For this review, use the dimensioned drawing (mm, ordinates from the lowest corner) and the shaded views. Coordinates: 2 decimals unless noted, no trailing zeros. Loops run counter-clockwise (first coordinate to the right, second up) from the corner with the lowest first, then second, coordinate; pieces in that order, holes last. Notation, with made-up numbers: (-4.75, -19) - (25.25, -19) arc R15 cw to (25.25, 0) - close; hole circle Ø5 at (42, -37). An arc over 180 degrees is marked (long way). Use a Markdown table: item, result. Add a question column.
1) Add section C-C, the plane y = 3.75. Give the boundary of the cut face in (x, z), and give its area (3 significant figures).
2) Add section A-A, the plane x = 44. Give the boundary of the cut face in (y, z), and give its area (3 significant figures).
3) The part is to be moulded in two halves that separate along Z. For the marked faces 1, 2 and 3, say which applies: pulls with the +Z half, pulls with the -Z half, needs draft (parallel to the pull), parting line crosses it, or undercut.
4) To check wall thickness, follow L1, parallel to X at y = 7.25, z = 9.75; L2, parallel to Z at x = 36, y = 3.5; L3, parallel to Z at x = 44, y = 3. State the ranges of each line that lie inside material, in increasing order. Write a range as [from, to].
5) Add section B-B, the plane z = 10. Give the boundary of the cut face in (x, y).
6) Add section D-D, the plane z = 6.5. Give the boundary of the cut face in (x, y).
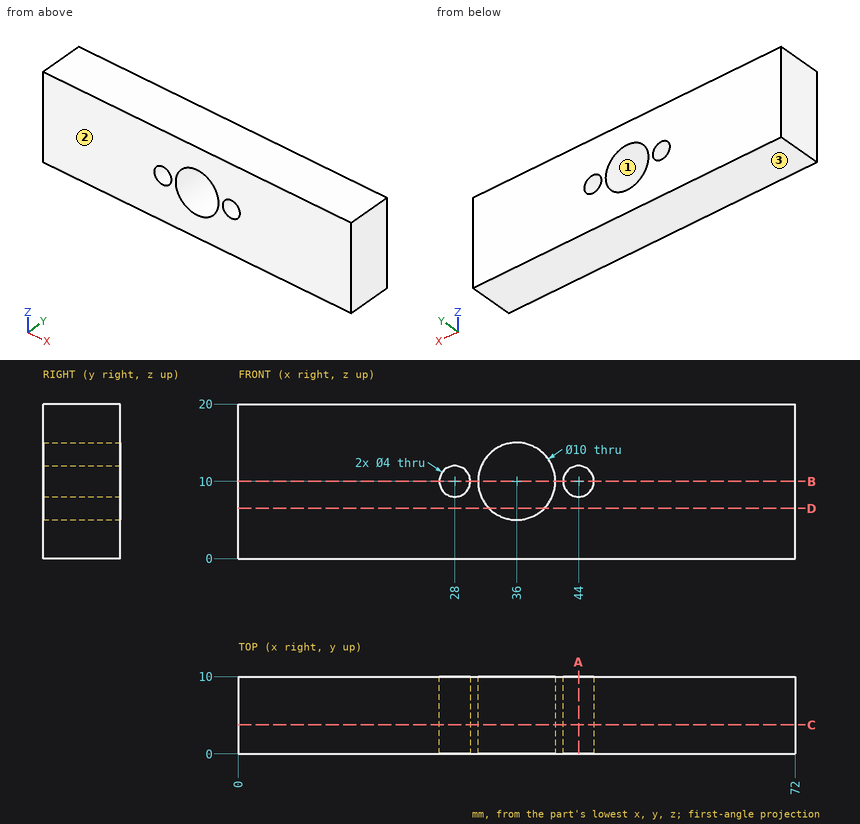
From the geometry:
| question | item | result |
|---|---|---|
| 1 | outline | (0, 0) - (72, 0) - (72, 20) - (0, 20) - close; hole circle Ø4 at (28, 10); hole circle Ø10 at (36, 10); hole circle Ø4 at (44, 10) |
| 1 | area | 1,340 mm^2 |
| 2 | outline | (0, 0) - (10, 0) - (10, 8) - (0, 8) - close; (0, 12) - (10, 12) - (10, 20) - (0, 20) - close |
| 2 | area | 160 mm^2 |
| 3 | face 1 | undercut |
| 3 | face 2 | needs draft |
| 3 | face 3 | pulls with the -Z half |
| 4 | L1 | x = [0, 26.02], [29.98, 31.01], [40.99, 42.02], [45.98, 72] |
| 4 | L2 | z = [0, 5], [15, 20] |
| 4 | L3 | z = [0, 8], [12, 20] |
| 5 | outline | (0, 0) - (26, 0) - (26, 10) - (0, 10) - close; (30, 0) - (31, 0) - (31, 10) - (30, 10) - close; (41, 0) - (42, 0) - (42, 10) - (41, 10) - close; (46, 0) - (72, 0) - (72, 10) - (46, 10) - close |
| 6 | outline | (0, 0) - (32.43, 0) - (32.43, 10) - (0, 10) - close; (39.57, 0) - (72, 0) - (72, 10) - (39.57, 10) - close |
